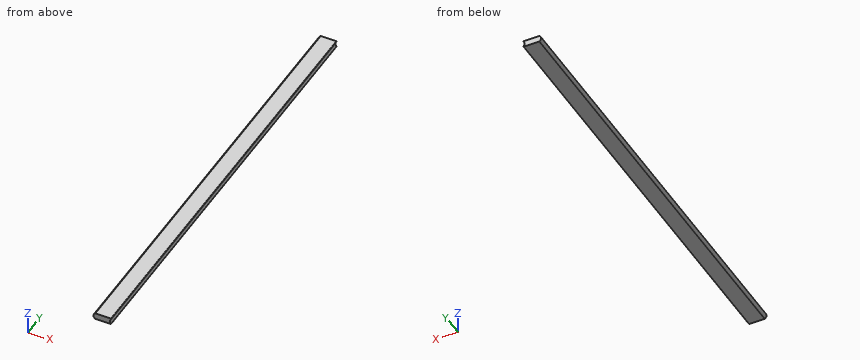
```python
from build123d import *

# Parameters (mm, degrees)
F0_W     = 100
F0_H     = 35
F1_DEPTH = 2400
F3_DEPTH = 2400


with BuildPart() as f1:
    # F0 (on Front) → F1 (new body)
    with BuildSketch(Plane.XZ):
        Rectangle(F0_W, F0_H)
    extrude(amount=F1_DEPTH)

    # F2 (on face) → F3 (cut, through all)
    with BuildSketch(Plane(origin=(0, 0, 0), x_dir=(-1, 0, 0), z_dir=(0, 1, 0))):
        with BuildLine():
            Line((-50, -17.5), (-47, -17.5))
            ThreePointArc((-47, -17.5), (-48.846372, -16.268706), (-48.419318, -14.090909))
            ThreePointArc((-48.419318, -14.090909), (-42.612495, 0), (-48.419318, 14.090909))
            ThreePointArc((-48.419318, 14.090909), (-48.846372, 16.268706), (-47, 17.5))
            Line((-47, 17.5), (-50, 17.5))
            Line((-50, 17.5), (-50, -17.5))
        make_face()
        with BuildLine():
            ThreePointArc((38.682458, 17.5), (49, 0), (38.682458, -17.5))
            Line((38.682458, -17.5), (50, -17.5))
            Line((50, -17.5), (50, 17.5))
            Line((50, 17.5), (38.682458, 17.5))
        make_face()
    extrude(amount=-F3_DEPTH, mode=Mode.SUBTRACT)


solid = f1.part
```
The model under review builds one solid part; all positions refer to its coordinate system, in mm. Give positions to 0.01 mm unless a question says otherwise; leave off trailing zeros. Write each loop counter-clockwise with the first axis right and the second up, starting at its lowest first coordinate (ties: lowest second). Pieces come first, ordered by that corner, then holes. Notation, with made-up numbers: M 18.5,44.5 L 48.5,44.5 A25 cw 48.5,80.5 Z; hole C 12,-26.75 d2. An arc over 180 degrees is marked long. Write item = value, one per line. Start each with the question number.
Q1. Clearance check with flat-ended pins moving along their axes: pin 1 (5 mm diameter, centred on y = -262, z = -4, fed in from +X); pin 2 (10 mm diameter, centred on y = -1352.5, z = 9, fed in from -X). State where each tip first meets the part, or that it passes through.
Q2. For line 1 (X direction, y = -1935, z = -2); line 2 (X direction, y = -926, z = 1); line 3 (Z direction, x = -42.5, y = -1059.5), list the stretches that pass through material, from the lowest coordinate up.
Q3. We need section B-B (z = -3.5). State the section outline as (x, y) points.
Q4. We need section A-A (y = -1034). State the section outline as (x, z) points, plus the area to 3 significant figures.
Result set:
q1.pin_1 = 43.7
q1.pin_2 = -48.6
q2.line_1 = -48.9 to 42.71
q2.line_2 = -48.97 to 42.64
q2.line_3 = -14.76 to 14.76
q3.outline = M -48.69,-2400 L 42.92,-2400 L 42.92,0 L -48.69,0 Z
q4.outline = M -38.68,-17.5 L 47,-17.5 A2 ccw 48.42,-14.09 A20 cw 48.42,14.09 A2 ccw 47,17.5 L -38.68,17.5 A20 ccw Z
q4.area = 3,190 mm2
